Input: part model. Units: mm. Frame: model coordinates. Face numbers are marked on the shaded views. A direction names the side the tool comes from. Coordinates: 2 decimals unless noted, no trailing zeros. Order: outer loops, then holes, each group sorted by start corner. A loop starts at its lowest first (then second) coordinate and runs counter-clockwise, first axis right, second up. Notation, with made-up numbers: (46, 39.5) - (101, 39.5) arc R20 cw to (101, 44.5) - close; hole circle Ø1 at (16, 49.25). An arc over 180 degrees is marked (long way). Answer as CSV lines item,"result". Start each with the question number.
Item 1: Section B-B (y = -216). Output: boundary loops of the cut face in (x, z).
Item 2: Section A-A (x = -37.5). Output: boundary loops of the cut face in (y, z), and give its area (3 significant figures).
Item 3: Section C-C (z = -432.5). Output: boundary loops of the cut face in (x, y), and give its area (3 significant figures).
Item 4: Draft query along Z for the marked faces 1, 2 and 3. Return one class per face: +Z half, -Z half, draft (parallel to the pull), parting line (faces both ways), or undercut.
Item 5: Material intervals for line 1 along Z through (x, y) = (-54, -227.5); line 2 along Z through (x, y) = (-124, -111.5); line 3 along Z through (x, y) = (186, -288), sorted ascending.
Item 6: Section D-D (x = -154). Output: boundary loops of the cut face in (y, z), and give its area (3 significant figures).
Item 7: First-contact query: pin 1 (8 mm diameter, centred on y = -121, z = -421.5, fed in from -X); pin 2 (10 mm diameter, centred on y = -217.5, z = -217.5, fed in from +X); pin 3 (2 mm diameter, centred on y = -155, z = -108.5, fed in from +X). Flat tips, straight axial feed; report the tip coordinate or a pass-through.
Item 8: Access query for the marked faces 4, 5 and 6. Directions: +Z, -Z, +X, -X, +Y, -Y. A direction counts if a zero-diameter tool reaches every point of the face in a straight line with its end or side. Return the directions, or none.
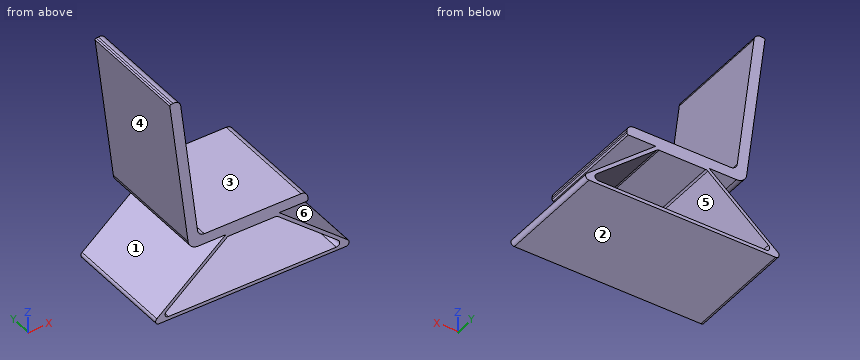
from build123d import *

# Parameters (mm, degrees)
F1_DEPTH = 406.4


with BuildPart() as f1:
    # F0 (on Front) → F1 (new body)
    with BuildSketch(Plane.XZ):
        with BuildLine():
            Line((-191.105931, -266.675295), (-228.921497, -271.322122))
            ThreePointArc((-228.921497, -271.322122), (-216.350395, -295.211711), (-191.105931, -304.775295))
            Line((-191.105931, -304.775295), (-191.105931, -266.675295))
        make_face()
        with BuildLine():
            Line((-193.846445, -244.37318), (-256.161501, 262.742624))
            ThreePointArc((-256.161501, 262.742624), (-265.735985, 279.661703), (-284.469762, 284.855116))
            Line((-284.469762, 284.855116), (-292.441746, 283.875508))
            ThreePointArc((-292.441746, 283.875508), (-295.551163, 282.115894), (-296.505617, 278.672969))
            Line((-296.505617, 278.672969), (-228.921497, -271.322122))
            Line((-228.921497, -271.322122), (-191.105931, -266.675295))
            Line((-191.105931, -266.675295), (-191.105931, -304.775295))
            Line((-191.105931, -304.775295), (-89.505931, -304.775295))
            Line((-89.505931, -304.775295), (108.589325, -304.775295))
            Line((108.589325, -304.775295), (210.189325, -304.775295))
            ThreePointArc((210.189325, -304.775295), (213.798924, -303.280151), (215.294069, -299.670552))
            Line((215.294069, -299.670552), (215.294069, -292.075295))
            ThreePointArc((215.294069, -292.075295), (207.854581, -274.114783), (189.894069, -266.675295))
            Line((189.894069, -266.675295), (-168.636068, -266.675295))
            ThreePointArc((-168.636068, -266.675295), (-185.46571, -260.299573), (-193.846445, -244.37318))
        make_face()
        with BuildLine():
            Line((108.589325, -304.775295), (-89.505931, -304.775295))
            Line((-89.505931, -304.775295), (-344.728743, -518.932662))
            ThreePointArc((-344.728743, -518.932662), (-348.499436, -533.005082), (-336.56534, -541.361427))
            Line((-336.56534, -541.361427), (355.648734, -541.361427))
            ThreePointArc((355.648734, -541.361427), (367.58283, -533.005082), (363.812136, -518.932662))
            Line((363.812136, -518.932662), (108.589325, -304.775295))
        make_face()
        with BuildLine():
            Line((-309.835779, -506.232662), (-84.880484, -317.472757))
            ThreePointArc((-84.880484, -317.472757), (-81.060737, -315.267425), (-76.717081, -314.501521))
            Line((-76.717081, -314.501521), (95.800475, -314.501521))
            ThreePointArc((95.800475, -314.501521), (100.144131, -315.267425), (103.963877, -317.472757))
            Line((103.963877, -317.472757), (328.919173, -506.232662))
            ThreePointArc((328.919173, -506.232662), (332.689867, -520.305082), (320.75577, -528.661427))
            Line((320.75577, -528.661427), (-301.672377, -528.661427))
            ThreePointArc((-301.672377, -528.661427), (-313.606473, -520.305082), (-309.835779, -506.232662))
        make_face(mode=Mode.SUBTRACT)
    extrude(amount=F1_DEPTH)


solid = f1.part
Determined:
1,outline,"(-344.73, -518.93) arc R12.7 ccw to (-336.57, -541.36) - (355.65, -541.36) arc R12.7 ccw to (363.81, -518.93) - (108.59, -304.78) - (210.19, -304.78) arc R5.1 ccw to (215.29, -299.67) - (215.29, -292.08) arc R25.4 ccw to (189.89, -266.68) - (-168.64, -266.68) arc R25.4 cw to (-193.85, -244.37) - (-256.16, 262.74) arc R25.4 ccw to (-284.47, 284.86) - (-292.44, 283.88) arc R4.67 ccw to (-296.51, 278.67) - (-228.92, -271.32) arc R38.1 ccw to (-191.11, -304.78) - (-89.51, -304.78) - close; hole (-309.84, -506.23) arc R12.7 ccw to (-301.67, -528.66) - (320.76, -528.66) arc R12.7 ccw to (328.92, -506.23) - (103.96, -317.47) arc R12.7 ccw to (95.8, -314.5) - (-76.72, -314.5) arc R12.7 ccw to (-84.88, -317.47) - close"
2,outline,"(-406.4, -541.36) - (0, -541.36) - (0, -528.66) - (-406.4, -528.66) - close; (-406.4, -314.5) - (0, -314.5) - (0, -266.68) - (-406.4, -266.68) - close"
2,area,"24,600 mm^2"
3,outline,"(-241.72, -406.4) - (-221.96, -406.4) - (-221.96, 0) - (-241.72, 0) - close; (241.05, -406.4) - (260.81, -406.4) - (260.81, 0) - (241.05, 0) - close"
3,area,"16,100 mm^2"
4,face 1,"undercut"
4,face 2,"-Z half"
4,face 3,"+Z half"
5,line 1,"z = -541.36 to -528.66, -314.5 to -266.68"
5,line 2,"z = -541.36 to -528.66, -350.3 to -333.72, -304.78 to -266.68"
5,line 3,"z = -541.36 to -528.66, -386.31 to -369.73, -304.78 to -266.68"
6,outline,"(-406.4, -541.36) - (0, -541.36) - (0, -528.66) - (-406.4, -528.66) - close; (-406.4, -375.47) - (0, -375.47) - (0, -358.89) - (-406.4, -358.89) - close; (-406.4, -304.78) - (0, -304.78) - (0, -266.68) - (-406.4, -266.68) - close"
6,area,"27,400 mm^2"
7,pin 1,"stops at x = -233.38"
7,pin 2,"stops at x = -196.53"
7,pin 3,"stops at x = -210.42"
8,face 4,"-X, +Y, -Y"
8,face 5,"+Y, -Y"
8,face 6,"+X, +Y, -Y"
